Verification items for the finished model (mm, model axes). A direction names the side the tool comes from. Give positions to 0.01 mm unless a question says otherwise; leave off trailing zeros. Loops run counter-clockwise (first coordinate to the right, second up) from the corner with the lowest first, then second, coordinate; pieces in that order, holes last. Notation, with made-up numbers: (50.5, 63) - (85.5, 63) arc R13 ccw to (85.5, 75) - close; hole circle Ø7 at (-39.5, -37). An arc over 180 degrees is marked (long way). One line per question, with ' | ' between items. Start each with the question number.
1. Section check A-A, the plane z = 0. Enter the section's corners in (x, y), then the cut area to 3 significant figures.
2. Section check B-B, the plane y = 4.5. Enter the section's corners in (x, z).
3. Tool access check on faces 4 (the face through (0.02, 2.46, -20.88)), 5 (the face through (3.7, 1, 0)), 6 (the face through (0, 5, -7)). Record the directions out of +Z, -Z, +X, -X, +Y, -Y that give a thin tool (end or side, any length) a straight path to the whole face; none if there is none.
4. Section check D-D, the plane z = 4. Enter the section's corners in (x, y).
5. Mould release check, pull along Z, two halves, no side actions. Record for faces 1 (the face through (2, 0, -4)), 2 (the face through (-1.08, 6.97, 4.88)), 3 (the face through (-2, 1.8, -2)): +Z half, -Z half, draft (parallel to the pull), parting line (faces both ways), or undercut.
6. Depth check by flat-ended pin: pin 1 Ø2 at (x, z) = (-1, -18) entering from -Y; pin 2 Ø2.5 at (x, z) = (0, 0) entering from -Y; pin 3 Ø1 at (x, y) = (4.5, 3.5) entering from +Z; pin 4 Ø1.5 at (y, z) = (3.5, -1.5) entering from +X. Enter the tip coordinate at first touch or a pass-through.
7. Section check C-C, the plane x = 1.25. Enter the section's corners in (y, z).
8. Thickness scan on line 1 along Z through (x, y) = (0, 7); line 2 along Y through (x, z) = (2.25, 2.5). Record the ranges inside material, lowest first. Write a range as from..to.
from build123d import *

# Parameters (mm, degrees)
BOSS_EXTRUDE2_DEPTH = 5
CUT_EXTRUDE1_REACH  = 7
SKETCH3_R           = 2.1
CUT_EXTRUDE3_DEPTH  = 1.8
SKETCH6_R           = 5
SKETCH6_R_2         = 2.1
BOSS_EXTRUDE3_DEPTH = 4


with BuildPart() as part:
    # Sketch1 → Boss-Extrude2 (new body)
    with BuildSketch(Plane(origin=(0, 0, 0), x_dir=(1, 0, 0), z_dir=(0, 1, 0))):
        with BuildLine():
            Line((-0.939692556, 20.223890242), (-7.329602442, 2.667757118))
            ThreePointArc((-7.329602442, 2.667757118), (0, -7.8), (7.329602442, 2.667757118))
            Line((7.329602442, 2.667757118), (0.939692556, 20.223890242))
            ThreePointArc((0.939692556, 20.223890242), (0, 20.881870053), (-0.939692556, 20.223890242))
        make_face()
    extrude(amount=BOSS_EXTRUDE2_DEPTH)

    # Sketch3 → Cut-Extrude1 (cut, up to next)
    with BuildSketch(Plane(origin=(0, 5, 0), x_dir=(1, 0, 0), z_dir=(0, 1, 0)), mode=Mode.PRIVATE) as cut_extrude1_sk1:
        Circle(SKETCH3_R)
    cut_extrude1_tool1 = extrude(cut_extrude1_sk1.sketch, amount=-CUT_EXTRUDE1_REACH, mode=Mode.PRIVATE) & part.part
    add(cut_extrude1_tool1.solids().sort_by_distance((0, 5, 0))[0], mode=Mode.SUBTRACT)

    # Sketch5 → Cut-Extrude3 (cut)
    with BuildSketch(Plane.XZ):
        Polygon((0, 4.272391992), (-3.7, 2.136195996), (-3.7, -2.136195996), (0, -4.272391992), (3.7, -2.136195996), (3.7, 2.136195996), align=None)
    extrude(amount=-CUT_EXTRUDE3_DEPTH, mode=Mode.SUBTRACT)

    # Sketch6 → Boss-Extrude3 (add)
    with BuildSketch(Plane(origin=(0, 5, 0), x_dir=(1, 0, 0), z_dir=(0, 1, 0))):
        Circle(SKETCH6_R)
        Circle(SKETCH6_R_2, mode=Mode.SUBTRACT)
    extrude(amount=BOSS_EXTRUDE3_DEPTH)


solid = part.part
Results list:
1) outline: (-7.8, 0) - (-3.7, 0) - (-3.7, 1.8) - (-2.1, 1.8) - (-2.1, 9) - (-5, 9) - (-5, 5) - (-7.8, 5) - close; (2.1, 1.8) - (3.7, 1.8) - (3.7, 0) - (7.8, 0) - (7.8, 5) - (5, 5) - (5, 9) - (2.1, 9) - close | area: 74.4 mm²
2) outline: (-7.33, -2.67) - (-0.94, -20.22) arc R1 ccw to (0.94, -20.22) - (7.33, -2.67) arc R7.8 ccw (long way) to start; hole circle Ø4.2 at (0, 0)
3) face 4: -Z, +Y, -Y | face 5: -Y | face 6: +Y
4) outline: (-6.7, 0) - (-0.47, 0) - (-0.47, 1.8) - (0.47, 1.8) - (0.47, 0) - (6.7, 0) - (6.7, 5) - (3, 5) - (3, 9) - (-3, 9) - (-3, 5) - (-6.7, 5) - close
5) face 1: draft | face 2: parting line | face 3: undercut
6) pin 1: y = 0 | pin 2: through | pin 3: z = 6.7 | pin 4: x = 7.76
7) outline: (0, -19.37) - (5, -19.37) - (5, -4.84) - (9, -4.84) - (9, -1.69) - (1.8, -1.69) - (1.8, -3.55) - (0, -3.55) - close; (0, 3.55) - (1.8, 3.55) - (1.8, 1.69) - (9, 1.69) - (9, 4.84) - (5, 4.84) - (5, 7.7) - (0, 7.7) - close
8) line 1: -5..-2.1, 2.1..5 | line 2: 1.8..9
